Design review of the part built by this model. Coordinates are the model's own, in mm. Face numbers are marked on the shaded views. A direction names the side the tool comes from. Coordinates: 2 decimals unless noted, no trailing zeros. Write each loop counter-clockwise with the first axis right and the second up, starting at its lowest first coordinate (ties: lowest second). Pieces come first, ordered by that corner, then holes. Notation, with made-up numbers: (44, -34.75) - (52, -34.75) arc R26 ccw to (52, 2.25) - close; hole circle Ø3 at (57, 85.25). An arc over 180 degrees is marked (long way). Use a Markdown table: item, result.
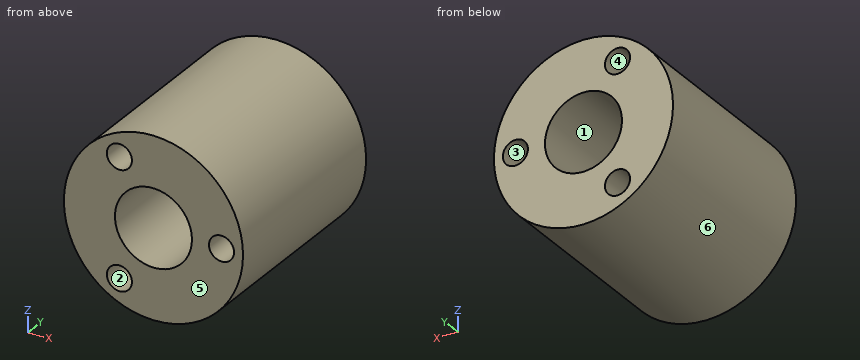
from build123d import *

# Parameters (mm, degrees)
SKETCH1_R           = 5
BOSS_EXTRUDE1_DEPTH = 5.5
SKETCH2_R           = 0.7
CUT_EXTRUDE1_DEPTH  = 2.5
HOLE1_START         = -5.5
HOLE1_OUTLINE_R     = 2.15
HOLE1_DEPTH         = 11


# Read off the part's stored shape, not the designer's step: Hole1
with BuildPart() as part:
    # Sketch1 → Boss-Extrude1 (new, symmetric)
    with BuildSketch(Plane(origin=(0, 0, 0), x_dir=(1, 0, 0), z_dir=(0, 1, 0))):
        with Locations(Location((0, 0, 0), (0, 0, 270))):
            Circle(SKETCH1_R)
    extrude(amount=BOSS_EXTRUDE1_DEPTH, both=True)

    # Sketch2 → Cut-Extrude1 (cut)
    with BuildSketch(Plane(origin=(0, 5.5, 0), x_dir=(1, 0, 0), z_dir=(0, 1, 0))):
        with Locations(Location((3.8, 0, 0), (0, 0, 270))):
            Circle(SKETCH2_R)
        with Locations(Location((-1.9, -3.290896534, 0), (0, 0, 270))):
            Circle(SKETCH2_R)
        with Locations(Location((-1.9, 3.290896534, 0), (0, 0, 270))):
            Circle(SKETCH2_R)
    cut_extrude1 = extrude(amount=-CUT_EXTRUDE1_DEPTH, mode=Mode.SUBTRACT)

    # Mirror1: Cut-Extrude1 across plane
    add(cut_extrude1.mirror(Plane.ZX), mode=Mode.SUBTRACT)

    # Hole1 outline → Hole1 (cut)
    with BuildSketch(Plane(origin=(0, 0, 0), x_dir=(1, 0, 0), z_dir=(0, 1, 0)).offset(HOLE1_START)):
        Circle(HOLE1_OUTLINE_R)
    extrude(amount=HOLE1_DEPTH, mode=Mode.SUBTRACT)


solid = part.part
(1) Machinability: for the marked faces 1, 2 and 3, which of the approach directions +Z, -Z, +X, -X, +Y, -Y give a long, thin tool a straight path to every point of the face, cutting with its end or side? Answer none if there is none.
Determined:
| item | result |
|---|---|
| face 1 | +Y, -Y |
| face 2 | -Y |
| face 3 | +Y |
(2) Take a section at C-C on y = -2.75. Write out the cut boundary in (x, z).
Determined:
| item | result |
|---|---|
| outline | circle Ø10 at (0, 0); hole circle Ø4.3 at (0, 0) |
(3) For L1, parallel to X at y = 4.8, z = 0; L2, parallel to X at y = 2.5, z = 0; L3, parallel to X at y = 4.25, z = 3.25, list the stretches that pass through material, from the lowest coordinate up. Write a range as from..to.
Determined:
| item | result |
|---|---|
| L1 | -5..-2.15, 2.15..3.1, 4.5..5 |
| L2 | -5..-2.15, 2.15..5 |
| L3 | -3.8..-2.6, -1.2..3.8 |
(4) Draft analysis for pull direction Z (two halves, no side actions). For the marked faces 4, 5 and 6, state which applies: +Z half, -Z half, draft (parallel to the pull), parting line (faces both ways), or undercut.
Determined:
| item | result |
|---|---|
| face 4 | undercut |
| face 5 | draft |
| face 6 | parting line |
(5) Take a section at A-A on z = 0. Write out the cut boundary in (x, y).
Determined:
| item | result |
|---|---|
| outline | (-5, -5.5) - (-2.15, -5.5) - (-2.15, 5.5) - (-5, 5.5) - close; (2.15, -5.5) - (3.1, -5.5) - (3.1, -3) - (4.5, -3) - (4.5, -5.5) - (5, -5.5) - (5, 5.5) - (4.5, 5.5) - (4.5, 3) - (3.1, 3) - (3.1, 5.5) - (2.15, 5.5) - close |
(6) Take a section at B-B on x = 0. Write out the cut boundary in (y, z), and give its area (3 significant figures).
Determined:
| item | result |
|---|---|
| outline | (-5.5, -5) - (5.5, -5) - (5.5, -2.15) - (-5.5, -2.15) - close; (-5.5, 2.15) - (5.5, 2.15) - (5.5, 5) - (-5.5, 5) - close |
| area | 62.7 mm2 |
(7) For pin 1 (1.5 mm diameter, centred on x = -1.5, z = -3.5, fed in from +Y); pin 2 (1.1 mm diameter, centred on x = -1.9, z = 3.29, fed in from +Y); pin 3 (0.7 mm diameter, centred on x = -2, z = -3, fed in from -Y); pin 4 (4 mm diameter, centred on y = 2, z = 3, fed in from -X), all flat-tipped, find the tip position at first contact; note any pin that passes through.
Determined:
| item | result |
|---|---|
| pin 1 | y = 5.5 |
| pin 2 | y = 3 |
| pin 3 | y = -3 |
| pin 4 | x = -4.9 |
(8) Take a section at D-D on z = -3.5. Write out the cut boundary in (x, y).
Determined:
| item | result |
|---|---|
| outline | (-3.57, -5.5) - (-2.57, -5.5) - (-2.57, -3) - (-1.23, -3) - (-1.23, -5.5) - (3.57, -5.5) - (3.57, 5.5) - (-1.23, 5.5) - (-1.23, 3) - (-2.57, 3) - (-2.57, 5.5) - (-3.57, 5.5) - close |
